Could you check a few things on this model? Use its own coordinates, in mm. A direction names the side the tool comes from. Give positions to 0.01 mm unless a question says otherwise; leave off trailing zeros. Write each loop counter-clockwise with the first axis right and the second up, starting at its lowest first coordinate (ties: lowest second). Pieces come first, ordered by that corner, then holes. Notation, with made-up numbers: (-18.5, 15) -> (-13.5, 15) arc R21 cw to (-13.5, 52) -> close; hole circle Ø3 at (-13.75, 76). An arc over 180 degrees is marked (long way). One line per question, with ' | ' between items.
Autodesk Inventor part; units mm, degrees
ref_plane "YZ Plane" through (0, 0, 0) normal (1, 0, 0) x (0, 1, 0)
ref_plane "XZ Plane" through (0, 0, 0) normal (0, 1, 0) x (-1, 0, 0)
ref_plane "XY Plane" through (0, 0, 0) normal (0, 0, 1) x (1, 0, 0)
sketch "スケッチ1" plane through (0, 0, 0) normal (0, 0, 1) x (1, 0, 0)
  line L0 (-35, 9.6) -> (-35, 16.25)
  line L1 (-35, 16.25) -> (-20, 16.25)
  line L2 (20, 16.25) -> (35, 16.25)
  line L3 (35, 16.25) -> (35, 9.6)
  line L4 (0, 0) -> (0, 16.25) construction
  line L5 (0, 0) -> (37, 0) construction
  line L6 (35, 7.5) -> (37, 7.5)
  line L7 (37, 7.5) -> (37, -7.5)
  line L8 (37, -7.5) -> (35, -7.5)
  line L9 (-20, -16.25) -> (20, -16.25) construction
  line L10 (20, -16.25) -> (20, 16.25) construction
  line L11 (20, 16.25) -> (-20, 16.25) construction
  line L12 (-20, 16.25) -> (-20, -16.25) construction
  line L13 (-20, -16.25) -> (20, 16.25) construction
  line L14 (20, -16.25) -> (-20, 16.25) construction
  line L15 (-35, -16.25) -> (35, -16.25) construction
  line L16 (35, -16.25) -> (35, 16.25) construction
  line L17 (35, 16.25) -> (-35, 16.25) construction
  line L18 (-35, 16.25) -> (-35, -16.25) construction
  line L19 (-35, -16.25) -> (35, 16.25) construction
  line L20 (35, -16.25) -> (-35, 16.25) construction
  arc A0 (35, 9.6) -> (35, 7.5) centre (35, 8.55) ccw
  arc A1 (35, -7.5) -> (35, -9.6) centre (35, -8.55) ccw
  line L21 (35, -9.6) -> (35, -16.25)
  line L22 (35, -16.25) -> (20, -16.25)
  line L23 (20, -16.25) -> (12.1, -16.25)
  line L24 (-20, 16.25) -> (-12.1, 16.25)
  line L25 (-10, 16.25) -> (-10, 18.25)
  line L26 (-10, 18.25) -> (10, 18.25)
  line L27 (10, 18.25) -> (10, 16.25)
  line L28 (20, 16.25) -> (12.1, 16.25)
  arc A2 (-12.1, 16.25) -> (-10, 16.25) centre (-11.05, 16.25) ccw
  arc A3 (10, 16.25) -> (12.1, 16.25) centre (11.05, 16.25) ccw
  line L29 (-35, 7.5) -> (-37, 7.5)
  line L30 (-37, 7.5) -> (-37, -7.5)
  line L31 (-37, -7.5) -> (-35, -7.5)
  arc A4 (-35, 7.5) -> (-35, 9.6) centre (-35, 8.55) ccw
  arc A5 (-35, -9.6) -> (-35, -7.5) centre (-35, -8.55) ccw
  line L32 (-35, -9.6) -> (-35, -16.25)
  line L33 (-35, -16.25) -> (-20, -16.25)
  line L34 (-20, -16.25) -> (-12.1, -16.25)
  line L35 (-10, -16.25) -> (-10, -18.25)
  line L36 (-10, -18.25) -> (10, -18.25)
  line L37 (10, -18.25) -> (10, -16.25)
  arc A6 (-10, -16.25) -> (-12.1, -16.25) centre (-11.05, -16.25) ccw
  arc A7 (12.1, -16.25) -> (10, -16.25) centre (11.05, -16.25) ccw
  line L38 (-16.55, 19.1799) -> (-13.45, 19.1799) construction
  line L39 (-13.45, 19.1799) -> (-13.45, 12.4242) construction
  line L40 (-13.45, 12.4242) -> (-16.55, 12.4242) construction
  line L41 (-16.55, 12.4242) -> (-16.55, 19.1799) construction
  line L42 (-15, 19.1799) -> (-15, 12.4242) construction
  point P0 (0, 18.25)
  point P1 (0, 0)
  dimension "d0" = 1.05
  dimension "d1" = 32.5
  dimension "d2" = 70
  dimension "d3" = 40
  dimension "d23" = 2
  dimension "d30" = 2
  dimension "d34" = 8.75
  dimension "d53" = 20
  dimension "d54" = 3.1
  dimension "d55" = 5
  dimension "d85" = 32.5
extrude "押し出し1" add sketch "スケッチ1" along normal blind 5
sketch "スケッチ2" plane through (0, 0, 0) normal (0, 0, -1) x (-1, 0, 0)
  line L0 (35, 9.6) -> (35, 16.25)
  line L1 (-35, 16.25) -> (-35, 9.6)
  line L2 (-43.1427, 17.3125) -> (-35, 17.3125)
  line L3 (-35, 17.3125) -> (-35, -16.751)
  line L4 (-35, -16.751) -> (-43.1427, -16.751)
  line L5 (-43.1427, -16.751) -> (-43.1427, 17.3125)
  line L6 (35, 21.1805) -> (40.858, 21.1805)
  line L7 (40.858, 21.1805) -> (40.858, -13.6193)
  line L8 (40.858, -13.6193) -> (35, -13.6193)
  line L9 (35, -13.6193) -> (35, 21.1805)
  line L10 (-20, -16.25) -> (-12.1, -16.25)
  line L11 (-17.1371, 25.1848) -> (11.8342, 25.1848)
  line L12 (11.8342, 25.1848) -> (11.8342, 16.25)
  line L13 (11.8342, 16.25) -> (-17.1371, 16.25)
  line L14 (-17.1371, 16.25) -> (-17.1371, 25.1848)
  line L15 (-13.151, -21.5857) -> (17.7795, -21.5857)
  line L16 (17.7795, -21.5857) -> (17.7795, -16.25)
  line L17 (17.7795, -16.25) -> (-13.151, -16.25)
  line L18 (-13.151, -16.25) -> (-13.151, -21.5857)
  line L19 (-12.1, 16.25) -> (-35, 16.25)
  line L20 (-35, -16.25) -> (-12.1, -16.25)
  point P0 (0, 0)
extrude "押し出し2" cut sketch "スケッチ2" against normal blind 2.5
sketch "スケッチ3" plane through (12.1, 16.25, 0) normal (0, 1, 0) x (1, 0, 0)
  line L0 (-2.1, 0) -> (-2.1, -5)
  line L1 (-2.1, -5) -> (-22.1, -5) construction
  line L2 (-12.1, -5) -> (-12.1, 7.4607) construction
  line L3 (22.9, 0) -> (22.9, -5)
  point P0 (-12.1, 0)
  point P1 (2.9, -2.5)
  point P2 (-27.1, -2.5)
  point P3 (22.9, -2.5)
  dimension "d60" = 5
hole "穴1" at (15, 16.25, 2.5) at (-15, 16.25, 2.5) direction (0, -1, 0) diameter 2.459 depth 2.5
mirror "ミラー1" about plane through (0, 0, 0) normal (0, 1, 0) of "穴1"
sketch "スケッチ4" plane through (35, -16.25, 5) normal (1, 0, 0) x (0, 0, -1)
  line L0 (5, 16.25) -> (0, 16.25) construction
  line L1 (0, 23.75) -> (0, 8.75) construction
  line L2 (5, 6.65) -> (0, 6.65)
  line L3 (5, 0) -> (0, 0)
  point P0 (2.5, 3)
  point P1 (2.5, 29.5)
  point P2 (2.5, 6.65)
  dimension "d86" = 3
  dimension "d87" = 26.5
hole "穴2" at (35, -13.25, 2.5) at (35, 13.25, 2.5) direction (-1, 0, 0) diameter 2.459 depth 2.5
mirror "ミラー2" about plane through (0, 0, 0) normal (1, 0, 0) of "穴2"
sketch "スケッチ5" plane through (0, 0, 0) normal (0, 0, -1) x (-1, 0, 0)
  line L0 (10, 16.25) -> (-10, 16.25)
  line L1 (-35, 7.5) -> (-35, 9.6)
  line L2 (-30, -11.25) -> (30, -11.25) construction
  line L3 (30, -11.25) -> (30, 11.25) construction
  line L4 (30, 11.25) -> (-30, 11.25) construction
  line L5 (-30, 11.25) -> (-30, -11.25) construction
  line L6 (-30, -11.25) -> (30, 11.25) construction
  line L7 (30, -11.25) -> (-30, 11.25) construction
  line L8 (-30, 9.114) -> (-30, -9.114)
  line L9 (-30, -9.114) -> (-5.696, 0)
  line L10 (-5.696, 0) -> (-30, 9.114)
  line L11 (-24.304, 11.25) -> (24.304, 11.25)
  line L12 (24.304, 11.25) -> (0, 2.136)
  line L13 (0, 2.136) -> (-24.304, 11.25)
  line L14 (-24.304, -11.25) -> (24.304, -11.25)
  line L15 (24.304, -11.25) -> (0, -2.136)
  line L16 (0, -2.136) -> (-24.304, -11.25)
  line L17 (30, 9.114) -> (30, -9.114)
  line L18 (30, -9.114) -> (5.696, 0)
  line L19 (5.696, 0) -> (30, 9.114)
  point P0 (-12.1, 16.25)
  point P1 (-20, 16.25)
  point P2 (-35, 16.25)
  point P3 (0, 0)
  dimension "d76" = 5
  dimension "d77" = 5
  dimension "d78" = 4
  dimension "d79" = 4
  dimension "d80" = 4
  dimension "d81" = 4
extrude "押し出し3" cut sketch "スケッチ5" against normal blind 10
fillet "フィレット1" radius 1.05 12 edges at (30, 9.114, 2.5) (30, -9.114, 2.5) (24.304, 11.25, 2.5) (5.696, 0, 2.5) (0, -2.136, 2.5) (0, 2.136, 2.5) (-30, -9.114, 2.5) (24.304, -11.25, 2.5) (-30, 9.114, 2.5) (-24.304, 11.25, 2.5) (-24.304, -11.25, 2.5) (-5.696, 0, 2.5)
equation "\"d85\" = d1"
equation "\"d77\" = d76"
equation "\"d79\" = d78"
equation "\"d80\" = d79"
equation "\"d81\" = d78"
equation "\"d52\" = 5"
properties part number "胴体_メインフレーム_1_13" material "アセタール樹脂、黒"
Q1. If I drill on line 1 along Y through (x, z) = (-33.9, 2.5); line 2 along X through (y, z) = (15.05, 2.5); line 3 along X through (y, z) = (15.45, 2.5), over which ranges is the centre line in solid material (lowest first)?
Answer below:
line 1: y = -16.25 to -14.48, -12.02 to 12.02, 14.48 to 16.25 | line 2: x = -35 to -16.23, -13.77 to 13.77, 16.23 to 35 | line 3: x = -35 to -16.23, -13.77 to -11.73, -10.37 to 10.37, 11.73 to 13.77, 16.23 to 35
Q2. Imagine slicing it at B-B on y = 5. Please give me the cut outline in (x, z).
Answer below:
outline: (-37, 2.5) -> (-35, 2.5) -> (-35, 0) -> (-30, 0) -> (-30, 5) -> (-37, 5) -> close; (-19.03, 0) -> (-7.64, 0) -> (-7.64, 5) -> (-19.03, 5) -> close; (7.64, 0) -> (19.03, 0) -> (19.03, 5) -> (7.64, 5) -> close; (30, 0) -> (35, 0) -> (35, 2.5) -> (37, 2.5) -> (37, 5) -> (30, 5) -> close
Q3. If we mould it in two halves opening along Z, with no side actions, what happens to faces 1 (the flat face through (32.5, -13, 3)), 2 (the cylindrical face through (-19.55, -10.37, 2.54)), 3 (the flat face through (0, -17, 2.5))? For each: +Z half, -Z half, draft (parallel to the pull), parting line (faces both ways), or undercut.
Answer below:
face 1: undercut | face 2: draft | face 3: -Z half
Q4. Imagine slicing it at A-A on x = 15. Please give me the cut outline in (y, z), and give its area (3 significant figures).
Answer below:
outline: (-16.25, 0) -> (-11.25, 0) -> (-11.25, 5) -> (-16.25, 5) -> (-16.25, 3.73) -> (-13.75, 3.73) -> (-13.75, 1.27) -> (-16.25, 1.27) -> close; (-7.76, 0) -> (-3.49, 0) -> (-3.49, 5) -> (-7.76, 5) -> close; (3.49, 0) -> (7.76, 0) -> (7.76, 5) -> (3.49, 5) -> close; (11.25, 0) -> (16.25, 0) -> (16.25, 1.27) -> (13.75, 1.27) -> (13.75, 3.73) -> (16.25, 3.73) -> (16.25, 5) -> (11.25, 5) -> close | area: 80.4 mm^2
Q5. On a 3-axis mill with a long thin cutter (end or side, diameter ignored), from which of +Z, -Z, +X, -X, +Y, -Y can I reach the whole of each face in a straight line? I mean faces 4 (the cylindrical face through (33.73, -14.47, 2.66)), 5 (the flat face through (9.5, 5.7, 2.5)), 6 (the flat face through (36, 7.5, 4)), 7 (the flat face through (0, 16.25, 1)). Say none if no direction works.
Answer below:
face 4: +X | face 5: +Z, -Z | face 6: +Z, -Z, +X, +Y | face 7: -Z, +X, -X, +Y
Q6. Imagine slicing it at D-D on x = -26.5. Please give me the cut outline in (y, z), and give its area (3 significant figures).
Answer below:
outline: (-16.25, 0) -> (-7.8, 0) -> (-7.8, 5) -> (-16.25, 5) -> close; (7.8, 0) -> (16.25, 0) -> (16.25, 5) -> (7.8, 5) -> close | area: 84.5 mm^2
Q7. Imagine slicing it at C-C on x = -4. Please give me the cut outline in (y, z).
Answer below:
outline: (-18.25, 2.5) -> (-16.25, 2.5) -> (-16.25, 0) -> (-11.25, 0) -> (-11.25, 5) -> (-18.25, 5) -> close; (-3.64, 0) -> (3.64, 0) -> (3.64, 5) -> (-3.64, 5) -> close; (11.25, 0) -> (16.25, 0) -> (16.25, 2.5) -> (18.25, 2.5) -> (18.25, 5) -> (11.25, 5) -> close
Q8. Will these pins go through, and if not, where does the flat tip stop? pin 1 (2 mm diameter, centred on y = -13.25, z = 2.5, fed in from +X); pin 2 (2 mm diameter, centred on x = -15, z = 2.5, fed in from -Y); pin 3 (2 mm diameter, centred on x = 35.5, y = 0.5, fed in from -Z); pin 4 (0.8 mm diameter, centred on x = 1.5, z = 1.5, fed in from +Y).
Answer below:
pin 1: stops at x = 32.5 | pin 2: stops at y = -13.75 | pin 3: stops at z = 0 | pin 4: stops at y = 16.25
